For this review, take the finished solid that the model builds, in its own axes (mm). A direction names the side the tool comes from. Give positions to 0.01 mm unless a question says otherwise; leave off trailing zeros. Loops run counter-clockwise (first coordinate to the right, second up) from the corner with the lowest first, then second, coordinate; pieces in that order, holes last. Notation, with made-up numbers: (25.5, 33) - (75.5, 33) arc R23 cw to (75.5, 61) - close; hole circle Ø8 at (88.25, -14). An arc over 180 degrees is marked (long way). Put each result on its own line as item: value.
from build123d import *

# Parameters (mm, degrees)
SKETCH005_R     = 8
PAD003_DEPTH    = 5
SKETCH006_R     = 4
PAD004_DEPTH    = 12.5
SKETCH008_R     = 7
SKETCH008_R_2   = 4
POCKET002_DEPTH = 3
POCKET003_DEPTH = 15.5
CHAMFER_ANGLE   = 65
CHAMFER_SIZE    = 3.99


with BuildPart() as part:
    # Sketch005 → Pad003 (new body)
    with BuildSketch(Plane.XY):
        Circle(SKETCH005_R)
    extrude(amount=PAD003_DEPTH)

    # Sketch006 (on Face3 of Pad003) → Pad004 (join)
    with BuildSketch(Plane.XY.offset(5)):
        Circle(SKETCH006_R)
    extrude(amount=PAD004_DEPTH)

    # Sketch008 (on Face2 of Pad004) → Pocket002 (cut)
    with BuildSketch(Plane(origin=(0, 0, 0), x_dir=(1, 0, 0), z_dir=(0, 0, -1))):
        Circle(SKETCH008_R)
        Circle(SKETCH008_R_2, mode=Mode.SUBTRACT)
    extrude(amount=-POCKET002_DEPTH, mode=Mode.SUBTRACT)

    # Sketch007 (on Face5 of Pad004) → Pocket003 (cut)
    with BuildSketch(Plane.XY.offset(17.5)):
        with BuildLine():
            ThreePointArc((-0.5, 2.95804), (-2.12132, 2.12132), (-2.95804, 0.5))
            Line((-2.95804, 0.5), (-1.75, 0.5))
            Line((-1.75, 0.5), (-1.75, -0.5))
            Line((-1.75, -0.5), (-2.95804, -0.5))
            ThreePointArc((-2.95804, -0.5), (-2.12132, -2.12132), (-0.5, -2.95804))
            Line((-0.5, -2.95804), (-0.5, -1.75))
            Line((-0.5, -1.75), (0.5, -1.75))
            Line((0.5, -1.75), (0.5, -2.95804))
            ThreePointArc((0.5, -2.95804), (2.12132, -2.12132), (2.95804, -0.5))
            Line((2.95804, -0.5), (1.75, -0.5))
            Line((1.75, -0.5), (1.75, 0.5))
            Line((1.75, 0.5), (2.95804, 0.5))
            ThreePointArc((2.95804, 0.5), (2.12132, 2.12132), (0.5, 2.95804))
            Line((0.5, 2.95804), (0.5, 1.75))
            Line((0.5, 1.75), (-0.5, 1.75))
            Line((-0.5, 1.75), (-0.5, 2.95804))
        make_face()
    extrude(amount=-POCKET003_DEPTH, mode=Mode.SUBTRACT)

    # Chamfer
    chamfer_edges = [part.edges().sort_by_distance(p)[0] for p in [
        (-4, 0, 5),
    ]]
    chamfer_side = part.faces().sort_by_distance((-7.773726, 0, 5))[0]
    chamfer(chamfer_edges, length=CHAMFER_SIZE, angle=CHAMFER_ANGLE, reference=chamfer_side)


solid = part.part
1) Insertion check: pin 1 Ø0.6 at (x, z) = (2.5, 13.5) entering from +Y; pin 2 Ø1 at (y, z) = (-2, 11.5) entering from +X; pin 3 Ø1 at (y, z) = (2.5, 6.5) entering from +X. Each pin has a flat end and moves straight along its axis. Give the tip position at first contact, or say it passes through.
Geometry check:
pin 1: stops at y = 3.43
pin 2: stops at x = 4.86
pin 3: stops at x = 7.15
2) Take a section at C-C on z = 12.5. State the section outline as (x, y) points, and give its area (3 significant figures).
Geometry check:
outline: circle Ø8.99 at (0, 0); hole (-2.96, -0.5) arc R3 ccw to (-0.5, -2.96) - (-0.5, -1.75) - (0.5, -1.75) - (0.5, -2.96) arc R3 ccw to (2.96, -0.5) - (1.75, -0.5) - (1.75, 0.5) - (2.96, 0.5) arc R3 ccw to (0.5, 2.96) - (0.5, 1.75) - (-0.5, 1.75) - (-0.5, 2.96) arc R3 ccw to (-2.96, 0.5) - (-1.75, 0.5) - (-1.75, -0.5) - close
area: 40.1 mm²
3) For faces 1 (the face through (-0.5, 2, 10)), 2 (the face through (3, 3, 3)), 3 (the face through (0, 2, 17.5)), list the 3-axis set-ups (+Z, -Z, +X, -X, +Y, -Y) from which the entire face can be reached by the end or side of a thin tool; tool diameter is ignored.
Geometry check:
face 1: +Z
face 2: -Z
face 3: +Z, +X, -X, +Y, -Y
4) Wall thickness on line 1 (Y direction, x = 0, z = 0.7); line 2 (Y direction, x = 0, z = 2.4); line 3 (X direction, y = -2.25, z = 16.5): over which ranges is each line inside the solid? List them lowest first.
Geometry check:
line 1: y = -8 to -7, -4 to 4, 7 to 8
line 2: y = -8 to -7, -4 to -1.75, 1.75 to 4, 7 to 8
line 3: x = -3.31 to -1.98, -0.5 to 0.5, 1.98 to 3.31
5) Draft analysis for pull direction Y (two halves, no side actions). For faces 4 (the face through (2.1, -2.14, 9.86)), 5 (the face through (-0.867, -3.905, 15.501)), 6 (the face through (4, -6, 0)), state which applies: pulls with the +Y half, pulls with the -Y half, needs draft (parallel to the pull), parting line crosses it, or undercut.
Geometry check:
face 4: undercut
face 5: parting line crosses it
face 6: needs draft
6) Take a section at D-D on z = 10.5. State the section outline as (x, y) points.
Geometry check:
outline: circle Ø10.85 at (0, 0); hole (-2.96, -0.5) arc R3 ccw to (-0.5, -2.96) - (-0.5, -1.75) - (0.5, -1.75) - (0.5, -2.96) arc R3 ccw to (2.96, -0.5) - (1.75, -0.5) - (1.75, 0.5) - (2.96, 0.5) arc R3 ccw to (0.5, 2.96) - (0.5, 1.75) - (-0.5, 1.75) - (-0.5, 2.96) arc R3 ccw to (-2.96, 0.5) - (-1.75, 0.5) - (-1.75, -0.5) - close
